```python
from build123d import *

# Parameters (mm, degrees)
F0_R      = 6
F1_DEPTH  = 7
F2_R      = 4.75
F3_DEPTH  = 2
F4_R      = 6
F5_DEPTH  = 79
F6_R      = 4.75
F7_DEPTH  = 2
F8_R      = 6
F9_DEPTH  = 10
F10_SIZE  = 1.24999
F12_W     = 13
F12_H     = 10
F13_DEPTH = 1


# Not quite as in the source:
# - a fillet or chamfer is up to 0.001 mm smaller than in the source, because OpenCascade refuses the exact size


with BuildPart() as f1:
    # F0 (on Front) → F1 (new body)
    with BuildSketch(Plane.XZ):
        Circle(F0_R)
    extrude(amount=-F1_DEPTH)

    # F2 (on face) → F3 (join)
    with BuildSketch(Plane(origin=(0, 7, 0), x_dir=(-1, 0, 0), z_dir=(0, 1, 0))):
        Circle(F2_R)
    extrude(amount=F3_DEPTH)

    # F4 (on face) → F5 (join)
    with BuildSketch(Plane(origin=(0, 9, 0), x_dir=(-1, 0, 0), z_dir=(0, 1, 0))):
        Circle(F4_R)
    extrude(amount=F5_DEPTH)

    # F6 (on face) → F7 (join)
    with BuildSketch(Plane(origin=(0, 88, 0), x_dir=(-1, 0, 0), z_dir=(0, 1, 0))):
        Circle(F6_R)
    extrude(amount=F7_DEPTH)

    # F8 (on face) → F9 (join)
    with BuildSketch(Plane(origin=(0, 90, 0), x_dir=(-1, 0, 0), z_dir=(0, 1, 0))):
        Circle(F8_R)
    extrude(amount=F9_DEPTH)

    # F10 (size 1.25 in the source; OpenCascade refuses exactly that, so slightly less here)
    f10_edges = [f1.edges().sort_by_distance(p)[0] for p in [
        (6, 3.5, 0),
        (-6, 0, 0),
        (-6, 7, 0),
        (-6, 95, 0),
        (6, 90, 0),
        (6, 100, 0),
    ]]
    chamfer(f10_edges, length=F10_SIZE)

    # F12 (on offset) → F13 (cut)
    with BuildSketch(Plane.XY.offset(6)):
        with Locations((0, 17)):
            Rectangle(F12_W, F12_H)
    f13 = extrude(amount=-F13_DEPTH, mode=Mode.SUBTRACT)

    # F14: F13 across plane
    add(f13.mirror(Plane.XY), mode=Mode.SUBTRACT)


solid = f1.part
```
Input: part model. Units: mm. Frame: model coordinates. A direction names the side the tool comes from. Coordinates: 2 decimals unless noted, no trailing zeros. Write each loop counter-clockwise with the first axis right and the second up, starting at its lowest first coordinate (ties: lowest second). Pieces come first, ordered by that corner, then holes.
1) Set-up query: faces 1 (the flat face through (0, 100, 0)), 2 (the flat face through (-4, 9, -3)), 3 (the flat face through (0, 17, 5)), 4 (the cylindrical face through (6, 48, 0)), 5 (the flat face through (0, 17, -5)). Return all of +Z, -Z, +X, -X, +Y, -Y with unobstructed straight access to the full face (end or side cutting, diameter ignored); none if empty.
2) Mould query, pull axis Y, two halves, no side actions, for faces 6 (the cylindrical face through (-6, 3, 0)), 7 (the flat face through (0, 0, 0)), 8 (the cylindrical face through (-2.192, 88.986, -4.214)). Classes: pulls with the +Y half, pulls with the -Y half, needs draft (parallel to the pull), parting line crosses it, or undercut.
3) Material intervals for line 1 along Y through (x, z) = (3.5, -3.5); line 2 along Y through (x, z) = (5.25, 1.75); line 3 along X through (y, z) = (74, -0.25), sorted ascending.
4) Pin query (flat end, axial travel): pin 1 Ø1 at (x, z) = (5, 3) entering from +Y; pin 2 Ø0.8 at (x, z) = (1, -5.5) entering from -Y; pin 3 Ø2 at (x, y) = (1.5, 16) entering from +Z. Return the tip coordinate at first contact, or that it passes through.
5) Section A-A on y = 26.5. Output: boundary loops of the cut face in (x, z), and give its area (3 significant figures).
Check result:
1. face 1: +Z, -Z, +X, -X, +Y
1. face 2: none
1. face 3: +Z, +X, -X
1. face 4: +Y, -Y
1. face 5: -Z, +X, -X
2. face 6: needs draft
2. face 7: pulls with the -Y half
2. face 8: undercut
3. line 1: y = 0.2 to 6.8, 9 to 88, 90.2 to 99.8
3. line 2: y = 0.78 to 6.22, 9 to 88, 90.78 to 99.22
3. line 3: x = -5.99 to 5.99
4. pin 1: stops at y = 99.42
4. pin 2: stops at y = 0.44
4. pin 3: stops at z = 5
5. outline: circle Ø12 at (0, 0)
5. area: 113 mm2
